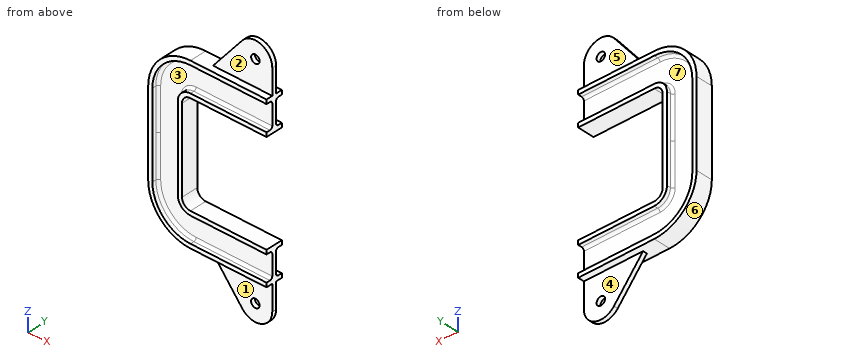
```python
from build123d import *

# Parameters (mm, degrees)
F4_R     = 5
F5_DEPTH = 2.5


with BuildPart() as f2:
    # F2: sweep along a path in F0
    with BuildLine(Plane.XZ) as f2_path:
        Line((0, 60), (-90, 60))
        ThreePointArc((-90, 60), (-97.071068, 57.071068), (-100, 50))
        Line((-100, 50), (-100, 0))
    # F1 (on Right) → F2 (sweep)
    with BuildSketch(Plane.YZ):
        with BuildLine():
            Line((10, 100), (0, 100))
            Line((0, 100), (-10, 100))
            Line((-10, 100), (-10, 95))
            Line((-10, 95), (-5.5, 95))
            ThreePointArc((-5.5, 95), (-3.37868, 94.12132), (-2.5, 92))
            Line((-2.5, 92), (-2.5, 68))
            ThreePointArc((-2.5, 68), (-3.37868, 65.87868), (-5.5, 65))
            Line((-5.5, 65), (-10, 65))
            Line((-10, 65), (-10, 60))
            Line((-10, 60), (0, 60))
            Line((0, 60), (10, 60))
            Line((10, 60), (10, 65))
            Line((10, 65), (5.5, 65))
            ThreePointArc((5.5, 65), (3.37868, 65.87868), (2.5, 68))
            Line((2.5, 68), (2.5, 92))
            ThreePointArc((2.5, 92), (3.37868, 94.12132), (5.5, 95))
            Line((5.5, 95), (10, 95))
            Line((10, 95), (10, 100))
        make_face()
    sweep(path=f2_path.line)

    # F3: F2 across plane


with BuildPart() as f2_1:
    add(f2.part)
    add(f2.part.mirror(Plane.XY))

    # F4 (on Front) → F5 (join, symmetric)
    with BuildSketch(Plane.XZ):
        with BuildLine():
            Line((0, -130), (0, -100))
            Line((0, -100), (-70, -100))
            Line((-70, -100), (-35.548045, -142.580075))
            ThreePointArc((-35.548045, -142.580075), (-13.327703, -148.854189), (0, -130))
        make_face()
        with Locations((-20, -130)):
            Circle(F4_R, mode=Mode.SUBTRACT)
    extrude(amount=F5_DEPTH, both=True)

    # F6: F2 across plane


with BuildPart() as f2_2:
    add(f2_1.part)
    add(f2_1.part.mirror(Plane.XY))


solid = f2_2.part
```
CAD build for the part. Positions are in the model's coordinates, mm. Face numbers are marked on the shaded views. A direction names the side the tool comes from. Round coordinates to 2 decimals unless told otherwise and drop trailing zeros. Write each loop counter-clockwise with the first axis right and the second up, starting at its lowest first coordinate (ties: lowest second). Pieces come first, ordered by that corner, then holes. Notation, with made-up numbers: M 34.25,-3 L 53.25,-3 A27 cw 53.25,33 Z; hole C 42,13 d7. An arc over 180 degrees is marked long. One line per question, with ' | ' between items.
1. Cut at B-B on z = -113. Write the cut outline in (x, y).
Working result:
outline: M -59.48,-2.5 L 0,-2.5 L 0,2.5 L -59.48,2.5 Z
2. Cut at A-A on x = -20. Count the separate pieces of the cut face and the enclosed holes in it, and give its area (3 significant figures).
Working result:
separate pieces: 4 | enclosed holes: 0 | area: 1,120 mm2
3. Probe L1, parallel to Z at x = -20, y = 0.3; L2, parallel to Z at x = -44, y = -6.5; L3, parallel to Y at x = -104.5, z = -82.5. List the from-to ranges inside material, lowest first. Write a range as from..to.
Working result:
L1: -150..-135, -125..-60, 60..125, 135..150 | L2: -100..-95, -65..-60, 60..65, 95..100 | L3: -2.5..2.5
4. Mould opens along Z. For the marked faces 5, 6 and 7 say: pulls with the +Z half, pulls with the -Z half, needs draft (parallel to the pull), parting line crosses it, or undercut.
Working result:
face 5: needs draft | face 6: pulls with the -Z half | face 7: undercut
5. Pin check, flat tips, straight feed: pin 1 Ø1.3 at (x, y) = (-40.5, 7) entering from -Z; pin 2 Ø12 at (y, z) = (-7.5, 42) entering from +X; pin 3 Ø3.5 at (x, y) = (-28, -8) entering from +Z. Stop position of each tip, or through.
Working result:
pin 1: z = -100 | pin 2: x = -100 | pin 3: z = 100
6. Which spindle directions (+Z, -Z, +X, -X, +Y, -Y) get a long thin tool onto all of the face, cutting with end or side? Do the marked faces 1, 2, 3 and 4. Say none if no direction does.
Working result:
face 1: -Z, +X, -X, -Y | face 2: +Z, +X, -X, -Y | face 3: -Y | face 4: -Z, +X, -X, +Y
